Part model, mm, in its own coordinate system. A direction names the side the tool comes from. Round coordinates to 2 decimals unless told otherwise and drop trailing zeros. Loops run counter-clockwise (first coordinate to the right, second up) from the corner with the lowest first, then second, coordinate; pieces in that order, holes last. Notation, with made-up numbers: (-33.5, -6) -> (10.5, -6) arc R17 cw to (10.5, 14) -> close; hole circle Ø4 at (15, 61). An arc over 180 degrees is marked (long way). Use a Markdown table: item, result. Add a question column.
Item 1: Which spindle directions (+Z, -Z, +X, -X, +Y, -Y) get a long thin tool onto all of the face, cutting with end or side? Do faces 1 (the face through (0, 0, 0)), 2 (the face through (38.69, 3.15, 0.7)). Say none if no direction does.
Item 2: Cut at D-D, the plane x = 9.5. List the corners of the cut face in (y, z), plus the area to 3 significant figures.
Item 3: Cut at A-A, the plane z = 0. List the corners of the cut face in (x, y) (3 decimals).
Item 4: Cut at C-C, the plane x = 47. List the corners of the cut face in (y, z) (3 decimals), plus the area to 3 significant figures.
Item 5: Probe line 1 (Y direction, x = 40.4, z = 0) (3 decimals); line 2 (Y direction, x = 38.05, z = 0) (3 decimals); line 3 (X direction, y = 4, z = -3). List the from-to ranges inside material, lowest first. Write a range as [from, to].
Item 6: Two-plate mould, pull along Y, no slides. Class faces 3 (the face through (50, 6, 0)), 4 (the face through (24.65, 7.509, -23.846)), 5 (the face through (42, 5, 0)): pulls with the +Y half, pulls with the -Y half, needs draft (parallel to the pull), parting line crosses it, or undercut.
Item 7: Flat gauge pins, fed straight in: pin 1 (8.5 mm diameter, centred on y = 0, z = 0, fed in from -X); pin 2 (10 mm diameter, centred on x = 26, z = -11.5, fed in from +Y); pin 3 (2 mm diameter, centred on x = 41, y = 17.5, fed in from -Z); pin 4 (8 mm diameter, centred on x = 33, y = -10.5, fed in from +Z). Where does each tip first touch, or does it go through?
```python
from build123d import *

# Parameters (mm, degrees)
SKETCH1_R           = 25
BOSS_EXTRUDE1_DEPTH = 50
SKETCH2_W           = 2.35
SKETCH2_H           = 3.225


with BuildPart() as part:
    # Sketch1 → Boss-Extrude1 (new body)
    with BuildSketch(Plane(origin=(0, 0, 0), x_dir=(0, 0, -1), z_dir=(1, 0, 0))):
        Circle(SKETCH1_R)
    extrude(amount=BOSS_EXTRUDE1_DEPTH)

    # Sketch2 → Cut-Revolve3 (revolve, cut)
    with BuildSketch(Plane(origin=(0, 0, 0), x_dir=(1, 0, 0), z_dir=(0, 1, 0))):
        Polygon((42, 0), (50, 0), (50, 5.275), (42, 5.275), (42, 4.675), align=None)
        Polygon((39.85, 0), (42, 0), (42, 4.675), (39.85, 4.675), (39.85, 3.225), align=None)
        with Locations((38.675, 1.6125)):
            Rectangle(SKETCH2_W, SKETCH2_H)
    revolve(axis=Axis((50, 0, 0), (-1, 0, 0)), mode=Mode.SUBTRACT)


solid = part.part
```
A:
| question | item | result |
|---|---|---|
| 1 | face 1 | +Z, -Z, -X, +Y, -Y |
| 1 | face 2 | +X |
| 2 | outline | circle Ø50 at (0, 0) |
| 2 | area | 1,960 mm^2 |
| 3 | outline | (0, -25) -> (50, -25) -> (50, -5.275) -> (42, -5.275) -> (42, -4.675) -> (39.85, -4.675) -> (39.85, -3.225) -> (37.5, -3.225) -> (37.5, 3.225) -> (39.85, 3.225) -> (39.85, 4.675) -> (42, 4.675) -> (42, 5.275) -> (50, 5.275) -> (50, 25) -> (0, 25) -> close |
| 4 | outline | circle Ø50 at (0, 0); hole circle Ø10.55 at (0, 0) |
| 4 | area | 1,880 mm^2 |
| 5 | line 1 | y = [-25, -4.675], [4.675, 25] |
| 5 | line 2 | y = [-25, -3.225], [3.225, 25] |
| 5 | line 3 | x = [0, 42] |
| 6 | face 3 | needs draft |
| 6 | face 4 | parting line crosses it |
| 6 | face 5 | undercut |
| 7 | pin 1 | stops at x = 0 |
| 7 | pin 2 | stops at y = 24.14 |
| 7 | pin 3 | stops at z = -18.78 |
| 7 | pin 4 | stops at z = 24.14 |
